Autodesk Inventor part; units mm, degrees
ref_plane "YZ Plane" through (0, 0, 0) normal (1, 0, 0) x (0, 1, 0)
ref_plane "XZ Plane" through (0, 0, 0) normal (0, 1, 0) x (-1, 0, 0)
ref_plane "XY Plane" through (0, 0, 0) normal (0, 0, 1) x (1, 0, 0)
sketch "Sketch1" plane through (0, 0, 0) normal (0, 1, 0) x (-1, 0, 0)
  line L0 (-44.45, 21.59) -> (44.45, 21.59)
  line L1 (44.45, 21.59) -> (44.45, -21.59)
  line L2 (44.45, -21.59) -> (-44.45, -21.59)
  line L3 (-44.45, -21.59) -> (-44.45, 21.59)
  line L4 (-44.45, 21.59) -> (44.45, -21.59) construction
  line L5 (44.45, 21.59) -> (-44.45, -21.59) construction
  point P0 (0, 0)
  dimension "d5" = 88.9
  dimension "d6" = 43.18
extrude "Extrusion1" add sketch "Sketch1" along normal blind 6.35
sketch "Sketch2" plane through (0, 6.35, 0) normal (0, 1, 0) x (1, 0, 0)
  line L0 (44.45, 21.59) -> (-44.45, 21.59)
  line L1 (44.45, -21.59) -> (44.45, 21.59)
  point P0 (0, 0)
  point P1 (0, -21.59)
  dimension "d16" = 43.18
  dimension "d17" = 44.45
hole "Hole1" at (0, 6.35, 21.59) direction (0, -1, 0) diameter 41.148 end through all
sketch "Sketch3" plane through (0, 6.35, 0) normal (0, 1, 0) x (1, 0, 0)
  line L0 (-44.45, 21.59) -> (-44.45, -21.59)
  line L1 (-44.45, -21.59) -> (-20.574, -21.59)
  point P0 (0, 0)
  point P1 (-31.75, -8.89)
  dimension "d25" = 12.7
  dimension "d26" = 12.7
hole "Hole2" at (-31.75, 6.35, 8.89) direction (0, -1, 0) diameter 4.826 end through all
sketch "Sketch4" plane through (0, 6.35, 0) normal (0, 1, 0) x (1, 0, 0)
  line L0 (44.45, 21.59) -> (-44.45, 21.59)
  line L1 (44.45, -21.59) -> (44.45, 21.59)
  point P0 (0, 0)
  point P1 (0, 8.89)
  dimension "d34" = 12.7
  dimension "d35" = 44.45
hole "Hole3" at (0, 6.35, -8.89) direction (0, -1, 0) diameter 4.826 end through all
sketch "Sketch5" plane through (0, 6.35, 0) normal (0, 1, 0) x (1, 0, 0)
  line L0 (44.45, -21.59) -> (44.45, 21.59)
  line L1 (20.574, -21.59) -> (44.45, -21.59)
  point P0 (0, 0)
  point P1 (31.75, -8.89)
  dimension "d43" = 12.7
  dimension "d44" = 12.7
hole "Hole4" at (31.75, 6.35, 8.89) direction (0, -1, 0) diameter 4.826 end through all
thread "Thread1"
thread "Thread2"
thread "Thread3"
properties part number "sguard"
Read the model definition and answer for the solid it produces. Units are mm, in the model's axes. Give positions to 0.01 mm unless a question says otherwise; leave off trailing zeros. Write each loop counter-clockwise with the first axis right and the second up, starting at its lowest first coordinate (ties: lowest second). Pieces come first, ordered by that corner, then holes. Notation, with made-up numbers: (77.5, -37) - (121.5, -37) arc R26 ccw to (121.5, -19) - close; hole circle Ø3 at (66, 75.25). An arc over 180 degrees is marked (long way). Return JSON: item names as keys, results as strings.
Q1. For a pull along X with two mould halves and no side action, classify faces 1 (the face through (44.45, 3, 0)), 2 (the face through (-29.394, 3.131, 8.367)), 3 (the face through (1, 6.35, -4)), 4 (the face through (-0.45, 3.13, 1.02)) as released by +X, released by -X, zero draft, split by the parting line, or undercut.
Reply:
{"face 1": "released by +X", "face 2": "undercut", "face 3": "zero draft", "face 4": "undercut"}
Q2. Consider line 1 along Z through (x, y) = (-31.75, 3); line 2 along X through (y, z) = (3.75, -8.89); line 3 along X through (y, z) = (4.5, 8.89). Determine where each line is inside the solid, lowest interval first. Write a range as [from, to].
Reply:
{"line 1": "[-21.59, 6.48], [11.3, 21.59]", "line 2": "[-44.45, -2.41], [2.41, 44.45]", "line 3": "[-44.45, -34.16], [-29.34, -16.19], [16.19, 29.34], [34.16, 44.45]"}
Q3. A cutting plane is placed at D-D, the plane z = 8.89. Determine the outline of the cut face in (x, y).
Reply:
{"outline": "(-44.45, 0) - (-34.16, 0) - (-34.16, 6.35) - (-44.45, 6.35) - close; (-29.34, 0) - (-16.19, 0) - (-16.19, 6.35) - (-29.34, 6.35) - close; (16.19, 0) - (29.34, 0) - (29.34, 6.35) - (16.19, 6.35) - close; (34.16, 0) - (44.45, 0) - (44.45, 6.35) - (34.16, 6.35) - close"}
Q4. A cutting plane is placed at A-A, the plane y = 5.5. Determine the outline of the cut face in (x, z).
Reply:
{"outline": "(-44.45, -21.59) - (44.45, -21.59) - (44.45, 21.59) - (20.57, 21.59) arc R20.57 cw to (-20.57, 21.59) - (-44.45, 21.59) - close; hole circle Ø4.83 at (-31.75, 8.89); hole circle Ø4.83 at (0, -8.89); hole circle Ø4.83 at (31.75, 8.89)"}
Q5. A cutting plane is placed at C-C, the plane z = -8.89. Determine the outline of the cut face in (x, y), and give its area (3 significant figures).
Reply:
{"outline": "(-44.45, 0) - (-2.41, 0) - (-2.41, 6.35) - (-44.45, 6.35) - close; (2.41, 0) - (44.45, 0) - (44.45, 6.35) - (2.41, 6.35) - close", "area": "534 mm²"}
Q6. Given P1, Ø3, axis at x = 16, y = 3, coming from the +Z side, flat-ended and moving along its own axis, determine where the tip first touches the part or whether it passes through.
Reply:
{"P1": "z = 10.77"}
Q7. A cutting plane is placed at B-B, the plane x = 0. Determine the outline of the cut face in (y, z).
Reply:
{"outline": "(0, -21.59) - (6.35, -21.59) - (6.35, -11.3) - (0, -11.3) - close; (0, -6.48) - (6.35, -6.48) - (6.35, 1.02) - (0, 1.02) - close"}
